Geometry check sheet. Reference: the model listing, model coordinates, mm. Face numbers are marked on the shaded views. A direction names the side the tool comes from. Give positions to 0.01 mm unless a question says otherwise; leave off trailing zeros. Loops run counter-clockwise (first coordinate to the right, second up) from the corner with the lowest first, then second, coordinate; pieces in that order, holes last. Notation, with made-up numbers: (9, 50) - (45, 50) arc R23 ccw to (45, 78) - close; hole circle Ø11 at (13, -4.5). An arc over 180 degrees is marked (long way). Use a Markdown table: item, result. Add a question column.
1. Draft check along Y on the marked faces 6, 7 and 8. Enter one of: pulls with the +Y half, pulls with the -Y half, needs draft (parallel to the pull), parting line crosses it, or undercut.
2. Depth check by flat-ended pin: P1, Ø2, axis at x = 34.5, y = 69.5, coming from the -Z side; P2, Ø8, axis at x = -24.5, z = -73.5, coming from the +Y side; P3, Ø3, axis at x = -21.5, z = 5.5, coming from the +Y side. Enter the tip coordinate at first touch or a pass-through.
3. Set-up check for the marked faces 1, 2, 3, 4 and 5: record each of +Z, -Z, +X, -X, +Y, -Y from which the full face is reachable in a straight line by a thin tool's end or side.
4. Cross-section at D-D on x = -5. Count the separate pieces of the cut face and the enclosed holes in it, and give its area (3 significant figures).
5. Material ranges on L1, parallel to X at y = 2, z = -3.5; L2, parallel to Y at x = 21.5, z = -44; L3, parallel to X at y = 76, z = 20, recorded low to high.
6. Cross-section at A-A on z = -73.5. Enter the section's corners in (x, y), and give its area (3 significant figures).
7. Cross-section at B-B on y = 49. Enter the section's corners in (x, z).
8. Cross-section at C-C on z = -11. Enter the section's corners in (x, y) (3 decimals), and give its area (3 significant figures).
from build123d import *

# Parameters (mm, degrees)
BOUNDARY2_START       = -200
BOUNDARY2_OUTLINE_W   = 78
BOUNDARY2_OUTLINE_H   = 48
BOUNDARY2_OUTLINE_W_2 = 72
BOUNDARY2_OUTLINE_H_2 = 42
BOUNDARY2_DEPTH       = 200
BOSS_EXTRUDE1_DEPTH   = 78
CUT_EXTRUDE7_DEPTH    = 72
SKETCH9_W             = 1
SKETCH9_H             = 83
BOSS_EXTRUDE2_DEPTH   = 78
SKETCH10_W            = 34
SKETCH10_H            = 83
BOSS_EXTRUDE3_DEPTH   = 3
SKETCH11_W            = 34
SKETCH11_H            = 83
BOSS_EXTRUDE4_DEPTH   = 3
SKETCH12_W            = 30
SKETCH12_H            = 30
CUT_EXTRUDE8_DEPTH    = 2
SKETCH13_R            = 1.5
CUT_EXTRUDE9_DEPTH    = 2
SKETCH14_W            = 30
SKETCH14_H            = 29.06458826
CUT_EXTRUDE10_DEPTH   = 45
CUT_EXTRUDE14_DEPTH   = 102
SKETCH19_W            = 64.171404934
SKETCH19_H            = 17.809337631
CUT_EXTRUDE15_DEPTH   = 102
SKETCH22_W            = 34
SKETCH22_H            = 3
BOSS_EXTRUDE5_DEPTH   = 4
SKETCH23_W            = 34
SKETCH23_H            = 3
BOSS_EXTRUDE6_DEPTH   = 4
IZIM1_W               = 78
IZIM1_H               = 48
IZIM1_W_2             = 72
IZIM1_H_2             = 42
KES_EKSTR_ZYON2_DEPTH = 105


# Read off the part's stored shape, not the designer's step: Boundary2
with BuildPart() as part:
    # Boundary2 outline → Boundary2 (new body)
    with BuildSketch(Plane.XY.offset(BOUNDARY2_START)):
        Rectangle(BOUNDARY2_OUTLINE_W, BOUNDARY2_OUTLINE_H)
        Rectangle(BOUNDARY2_OUTLINE_W_2, BOUNDARY2_OUTLINE_H_2, mode=Mode.SUBTRACT)
    extrude(amount=BOUNDARY2_DEPTH)

    # Sketch4 → Boss-Extrude1 (add)
    with BuildSketch(Plane.ZY.offset(39)):
        with BuildLine():
            Line((35, 31), (0, 31))
            Line((0, 31), (0, -24))
            ThreePointArc((0, -24), (25.621419403, -1.668175984), (35, 31))
        make_face()
    extrude(amount=-BOSS_EXTRUDE1_DEPTH)

    # Sketch7 → Cut-Extrude7 (cut)
    with BuildSketch(Plane(origin=(36, 0, 0), x_dir=(0, 0, -1), z_dir=(1, 0, 0))):
        with BuildLine():
            Line((-34, 31), (0, 31))
            Line((0, 31), (0, -21))
            ThreePointArc((0, -21), (-23.813697573, 0.544890049), (-34, 31))
        make_face()
    extrude(amount=-CUT_EXTRUDE7_DEPTH, mode=Mode.SUBTRACT)

    # Sketch9 → Boss-Extrude2 (add)
    with BuildSketch(Plane.ZY.offset(39)):
        with Locations((34.5, 72.5)):
            Rectangle(SKETCH9_W, SKETCH9_H)
    extrude(amount=-BOSS_EXTRUDE2_DEPTH)

    # Sketch10 → Boss-Extrude3 (add)
    with BuildSketch(Plane(origin=(39, 0, 0), x_dir=(0, 0, -1), z_dir=(1, 0, 0))):
        with Locations((-17, 72.5)):
            Rectangle(SKETCH10_W, SKETCH10_H)
    extrude(amount=-BOSS_EXTRUDE3_DEPTH)

    # Sketch11 → Boss-Extrude4 (add)
    with BuildSketch(Plane.ZY.offset(39)):
        with Locations((17, 72.5)):
            Rectangle(SKETCH11_W, SKETCH11_H)
    extrude(amount=-BOSS_EXTRUDE4_DEPTH)

    # Sketch12 → Cut-Extrude8 (cut)
    with BuildSketch(Plane.ZY.offset(-36)):
        with Locations((17, 89)):
            Rectangle(SKETCH12_W, SKETCH12_H)
    extrude(amount=-CUT_EXTRUDE8_DEPTH, mode=Mode.SUBTRACT)

    # Sketch13 → Cut-Extrude9 (cut)
    with BuildSketch(Plane.ZY.offset(-38)):
        with Locations((5, 101.5)):
            Circle(SKETCH13_R)
        with Locations((9, 101.5)):
            Circle(SKETCH13_R)
        with Locations((13, 101.5)):
            Circle(SKETCH13_R)
        with Locations((17, 101.5)):
            Circle(SKETCH13_R)
        with Locations((21, 101.5)):
            Circle(SKETCH13_R)
        with Locations((25, 101.5)):
            Circle(SKETCH13_R)
        with Locations((29, 101.5)):
            Circle(SKETCH13_R)
    extrude(amount=-CUT_EXTRUDE9_DEPTH, mode=Mode.SUBTRACT)

    # Sketch14 → Cut-Extrude10 (cut)
    with BuildSketch(Plane(origin=(0, 114, 0), x_dir=(1, 0, 0), z_dir=(0, 1, 0))):
        with Locations((0, -34)):
            Rectangle(SKETCH14_W, SKETCH14_H)
    extrude(amount=-CUT_EXTRUDE10_DEPTH, mode=Mode.SUBTRACT)

    # Sketch17 → Cut-Extrude14 (cut)
    with BuildSketch(Plane.ZY.offset(39)):
        Polygon((-100.968873407, 0), (-111.602076583, 18.417248148), (-132.868482935, 18.417248148), (-143.501686111, 0), (-132.868482935, -18.417248148), (-111.602076583, -18.417248148), align=None)
        Polygon((-149.750833218, 0), (-160.384036394, 18.417248148), (-181.650442746, 18.417248148), (-192.283645923, 0), (-181.650442746, -18.417248148), (-160.384036394, -18.417248148), align=None)
        Polygon((-52.186913596, 0), (-62.820116772, 18.417248148), (-84.086523124, 18.417248148), (-94.7197263, 0), (-84.086523124, -18.417248148), (-62.820116772, -18.417248148), align=None)
        Polygon((-3.404953785, 0), (-14.038156961, 18.417248148), (-35.304563313, 18.417248148), (-45.937766489, 0), (-35.304563313, -18.417248148), (-14.038156961, -18.417248148), align=None)
    extrude(amount=-CUT_EXTRUDE14_DEPTH, mode=Mode.SUBTRACT)

    # Sketch19 → Cut-Extrude15 (cut)
    with BuildSketch(Plane(origin=(0, 24, 0), x_dir=(1, 0, 0), z_dir=(0, 1, 0))):
        with Locations((0, 154.262884124)):
            Rectangle(SKETCH19_W, SKETCH19_H)
        with Locations((0, 179.262884124)):
            Rectangle(SKETCH19_W, SKETCH19_H)
        with Locations((0, 129.262884124)):
            Rectangle(SKETCH19_W, SKETCH19_H)
        with Locations((0, 104.262884124)):
            Rectangle(SKETCH19_W, SKETCH19_H)
        with Locations((0, 79.262884124)):
            Rectangle(SKETCH19_W, SKETCH19_H)
        with Locations((0, 54.262884124)):
            Rectangle(SKETCH19_W, SKETCH19_H)
        with Locations((0, 29.262884124)):
            Rectangle(SKETCH19_W, SKETCH19_H)
    extrude(amount=-CUT_EXTRUDE15_DEPTH, mode=Mode.SUBTRACT)

    # Sketch22 → Boss-Extrude5 (add)
    with BuildSketch(Plane(origin=(-36, 0, 0), x_dir=(0, 0, -1), z_dir=(1, 0, 0))):
        with Locations((-17, 112.5)):
            Rectangle(SKETCH22_W, SKETCH22_H)
    extrude(amount=BOSS_EXTRUDE5_DEPTH)

    # Sketch23 → Boss-Extrude6 (add)
    with BuildSketch(Plane.ZY.offset(-36)):
        with Locations((17, 112.5)):
            Rectangle(SKETCH23_W, SKETCH23_H)
    extrude(amount=BOSS_EXTRUDE6_DEPTH)

    # Çizim1 → Kes-Ekstrüzyon2 (cut)
    with BuildSketch(Plane(origin=(0, 0, -200), x_dir=(-1, 0, 0), z_dir=(0, 0, -1))):
        Rectangle(IZIM1_W, IZIM1_H)
        Rectangle(IZIM1_W_2, IZIM1_H_2, mode=Mode.SUBTRACT)
    extrude(amount=-KES_EKSTR_ZYON2_DEPTH, mode=Mode.SUBTRACT)


solid = part.part
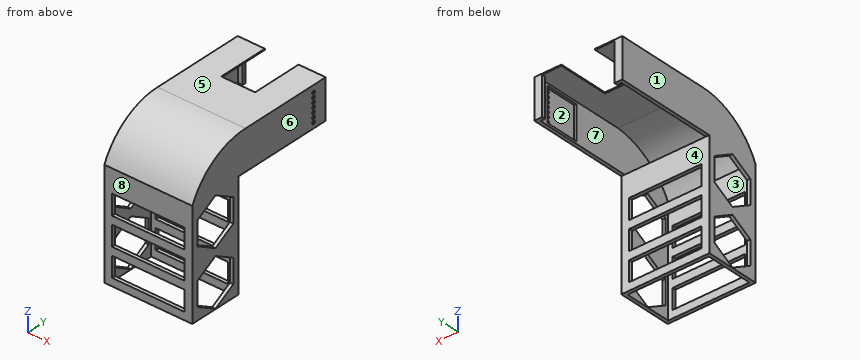
Values found:
| question | item | result |
|---|---|---|
| 1 | face 6 | needs draft |
| 1 | face 7 | undercut |
| 1 | face 8 | pulls with the -Y half |
| 2 | P1 | stops at z = 34 |
| 2 | P2 | stops at y = 24 |
| 2 | P3 | stops at y = -16.77 |
| 3 | face 1 | +Z, -Z, -X, +Y, -Y |
| 3 | face 2 | none |
| 3 | face 3 | -Z |
| 3 | face 4 | -Z, +X, -X, +Y |
| 3 | face 5 | +Z, +X, -X, +Y, -Y |
| 4 | separate pieces | 8 |
| 4 | enclosed holes | 0 |
| 4 | area | 450 mm2 |
| 5 | L1 | x = -39 to -36, 36 to 39 |
| 5 | L2 | y = -24 to -21, 21 to 24 |
| 5 | L3 | x = -39 to -36, 38 to 39 |
| 6 | outline | (-39, -24) - (-32.09, -24) - (-32.09, -21) - (-36, -21) - (-36, -18.42) - (-39, -18.42) - close; (-39, 18.42) - (-36, 18.42) - (-36, 21) - (-32.09, 21) - (-32.09, 24) - (-39, 24) - close; (32.09, -24) - (39, -24) - (39, -18.42) - (36, -18.42) - (36, -21) - (32.09, -21) - close; (32.09, 21) - (36, 21) - (36, 18.42) - (39, 18.42) - (39, 24) - (32.09, 24) - close |
| 6 | area | 114 mm2 |
| 7 | outline | (-39, 0) - (-36, 0) - (-36, 34) - (36, 34) - (36, 0) - (39, 0) - (39, 35) - (-39, 35) - close |
| 8 | outline | (-39, -24) - (39, -24) - (39, -13.155) - (36, -13.155) - (36, -21) - (-36, -21) - (-36, -13.155) - (-39, -13.155) - close; (-39, 13.155) - (-36, 13.155) - (-36, 21) - (36, 21) - (36, 13.155) - (39, 13.155) - (39, 24) - (-39, 24) - close |
| 8 | area | 562 mm2 |
